Here's how the part is built. I have some questions about the finished solid (model axes, mm). Face numbers are marked on the shaded views. Round coordinates to 2 decimals unless told otherwise and drop trailing zeros. Order: outer loops, then holes, each group sorted by start corner. A loop starts at its lowest first (then second) coordinate and runs counter-clockwise, first axis right, second up. Notation, with made-up numbers: (-23.75, 59.5) -> (1.25, 59.5) arc R16 ccw to (1.25, 87.5) -> close; hole circle Ø7 at (-24, 18). An arc over 180 degrees is marked (long way). Answer in a Markdown table with one row per item.
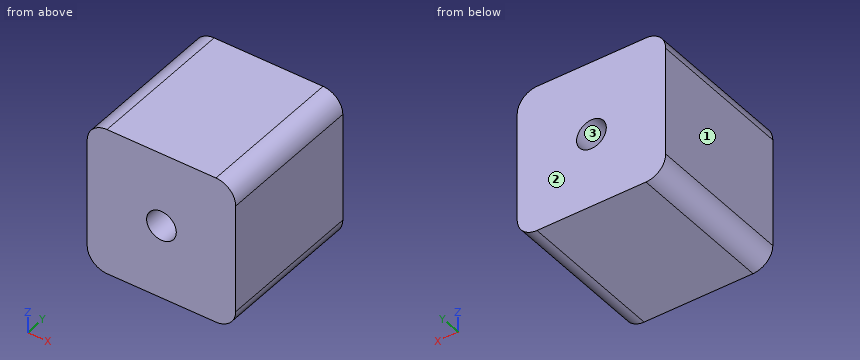
```python
from build123d import *

# Parameters (mm, degrees)
F1_DEPTH = 150
F2_R     = 15
F3_DEPTH = 150.001


with BuildPart() as f1:
    # F0 (on Front) → F1 (new body)
    with BuildSketch(Plane.XZ):
        with BuildLine():
            Line((55, 75), (-55, 75))
            ThreePointArc((-55, 75), (-69.142136, 69.142136), (-75, 55))
            Line((-75, 55), (-75, -55))
            ThreePointArc((-75, -55), (-69.142136, -69.142136), (-55, -75))
            Line((-55, -75), (55, -75))
            ThreePointArc((55, -75), (69.142136, -69.142136), (75, -55))
            Line((75, -55), (75, 55))
            ThreePointArc((75, 55), (69.142136, 69.142136), (55, 75))
        make_face()
    extrude(amount=F1_DEPTH)

    # F2 (on face) → F3 (cut, through all)
    with BuildSketch(Plane.XZ.offset(150)):
        Circle(F2_R)
    extrude(amount=-F3_DEPTH, mode=Mode.SUBTRACT)


solid = f1.part
```
1. Suppose I cut it at C-C on y = -87. Write out the boundary of the cut face in (x, z).
Numbers:
| item | result |
|---|---|
| outline | (-75, -55) arc R20 ccw to (-55, -75) -> (55, -75) arc R20 ccw to (75, -55) -> (75, 55) arc R20 ccw to (55, 75) -> (-55, 75) arc R20 ccw to (-75, 55) -> close; hole circle Ø30 at (0, 0) |
2. Please list where these lines run through material, in increasing order: line 1 along Z through (x, y) = (0, -83.5); line 2 along Z through (x, y) = (-3, -44); line 3 along X through (y, z) = (-115, 9).
Numbers:
| item | result |
|---|---|
| line 1 | z = -75 to -15, 15 to 75 |
| line 2 | z = -75 to -14.7, 14.7 to 75 |
| line 3 | x = -75 to -12, 12 to 75 |
3. Suppose I cut it at B-B on x = 0. Write out the boundary of the cut face in (y, z), then the cut area to 3 significant figures.
Numbers:
| item | result |
|---|---|
| outline | (-150, -75) -> (0, -75) -> (0, -15) -> (-150, -15) -> close; (-150, 15) -> (0, 15) -> (0, 75) -> (-150, 75) -> close |
| area | 18,000 mm2 |
4. Suppose I cut it at A-A on z = 0. Write out the boundary of the cut face in (x, y).
Numbers:
| item | result |
|---|---|
| outline | (-75, -150) -> (-15, -150) -> (-15, 0) -> (-75, 0) -> close; (15, -150) -> (75, -150) -> (75, 0) -> (15, 0) -> close |
5. We'd pull the mould along X, two halves only. Please class the marked faces 1, 2 and 3: released by +X, released by -X, zero draft, split by the parting line, or undercut.
Numbers:
| item | result |
|---|---|
| face 1 | released by -X |
| face 2 | zero draft |
| face 3 | undercut |
